Geometry check sheet. Reference: the model listing, model coordinates, mm. Face numbers are marked on the shaded views. A direction names the side the tool comes from. Coordinates: 2 decimals unless noted, no trailing zeros. Write each loop counter-clockwise with the first axis right and the second up, starting at its lowest first coordinate (ties: lowest second). Pieces come first, ordered by that corner, then holes. Notation, with made-up numbers: (17, -32.75) -> (51, -32.75) arc R16 ccw to (51, -27.75) -> close; hole circle Ø7 at (-3.75, 45). An arc over 180 degrees is marked (long way). Answer in a Markdown table with one row per item. Add a question column.
Q1. Release check for a two-part mould opening along Z. For the marked faces 1, 2, 3 and 4 record: pulls with the +Z half, pulls with the -Z half, needs draft (parallel to the pull), parting line crosses it, or undercut.
Q2. Tool access check on the marked faces 5 and 6. Record the directions out of +Z, -Z, +X, -X, +Y, -Y that give a thin tool (end or side, any length) a straight path to the whole face; none if there is none.
Q3. Section check B-B, the plane x = 11. Record the boundary of the cut face in (y, z), and give its area (3 significant figures).
Q4. Section check A-A, the plane z = -12. Record the boundary of the cut face in (x, y).
Q5. Gauge pin test, flat ends, axial feed: P1, Ø3, axis at x = -28.47, z = 35.745, coming from the +Y side; P2, Ø10, axis at x = -21, z = -12.5, coming from the +Y side; P3, Ø2, axis at x = -67.11, z = -42.11, coming from the +Y side. Record the tip position at first contact, or that the pin passes through.
Q6. Thickness scan on line 1 (Z direction, x = -28.47, y = 8) (3 decimals); line 2 (Z direction, x = -32.5, y = 26.75); line 3 (X direction, y = 24.5, z = 1.5). Record the ranges inside material, lowest first.
```python
from build123d import *

# Parameters (mm, degrees)
SKETCH1_W                 = 150
SKETCH1_H                 = 100
BOSS_EXTRUDE1_DEPTH       = 10
SKETCH2_R                 = 2.75
BOSS_EXTRUDE2_DEPTH       = 3
F_1_0MM_DOWEL_HOLE1_D     = 2.6
F_1_0MM_DOWEL_HOLE1_DEPTH = 10
F_1_0MM_DOWEL_HOLE1_TIP   = 0.781118805
FILLET1_R                 = 2
SKETCH5_W                 = 150
SKETCH5_H                 = 25
BOSS_EXTRUDE3_DEPTH       = 10
SKETCH7_W                 = 150
SKETCH7_H                 = 125
SKETCH7_W_2               = 136
SKETCH7_H_2               = 111
EXTRUDE_THIN1_DEPTH       = 20
CUT_EXTRUDE1_REACH        = 150.829
FILLET2_R                 = 15
FILLET3_R                 = 15
SKETCH9_R                 = 1.725
CUT_EXTRUDE2_DEPTH        = 6


with BuildPart() as part:
    # Sketch1 → Boss-Extrude1 (new body)
    with BuildSketch(Plane(origin=(0, 0, 0), x_dir=(1, 0, 0), z_dir=(0, 1, 0))):
        Rectangle(SKETCH1_W, SKETCH1_H)
    extrude(amount=BOSS_EXTRUDE1_DEPTH)

    # Sketch2 → Boss-Extrude2 (add)
    with BuildSketch(Plane(origin=(0, 10, 0), x_dir=(1, 0, 0), z_dir=(0, 1, 0))):
        with Locations(Location((28.47, 35.745, 0), (0, 0, 270))):
            Circle(SKETCH2_R)
        with Locations(Location((28.47, -35.745, 0), (0, 0, 90))):
            Circle(SKETCH2_R)
        with Locations(Location((-28.47, -35.745, 0), (0, 0, 270))):
            Circle(SKETCH2_R)
        with Locations(Location((-28.47, 35.745, 0), (0, 0, 90))):
            Circle(SKETCH2_R)
    extrude(amount=BOSS_EXTRUDE2_DEPTH)

    # Ø1.0mm Dowel Hole1
    with Locations(Plane(origin=(0, 13, 0), x_dir=(1, 0, 0), z_dir=(0, 1, 0))):
        with Locations((-28.47, 35.745), (28.47, 35.745), (28.47, -35.745), (-28.47, -35.745)):
            Hole(F_1_0MM_DOWEL_HOLE1_D / 2, depth=F_1_0MM_DOWEL_HOLE1_DEPTH)
            with Locations((0, 0, -(F_1_0MM_DOWEL_HOLE1_DEPTH + F_1_0MM_DOWEL_HOLE1_TIP / 2))):  # 118° drill point
                Cone(0, F_1_0MM_DOWEL_HOLE1_D / 2, F_1_0MM_DOWEL_HOLE1_TIP, mode=Mode.SUBTRACT)

    # Fillet1
    fillet1_edges = [part.edges().sort_by_distance(p)[0] for p in [
        (-28.47, 10, 32.995),
        (28.47, 10, -38.495),
        (28.47, 10, 38.495),
        (-28.47, 10, -32.995),
    ]]
    fillet(fillet1_edges, radius=FILLET1_R)

    # Sketch5 → Boss-Extrude3 (add)
    with BuildSketch(Plane.XZ):
        with Locations((0, 62.5)):
            Rectangle(SKETCH5_W, SKETCH5_H)
    extrude(amount=-BOSS_EXTRUDE3_DEPTH)

    # Sketch7 → Extrude-Thin1 (add)
    with BuildSketch(Plane(origin=(0, 10, 0), x_dir=(1, 0, 0), z_dir=(0, 1, 0))):
        with Locations((0, -12.5)):
            Rectangle(SKETCH7_W, SKETCH7_H)
        with Locations((0, -12.5)):
            Rectangle(SKETCH7_W_2, SKETCH7_H_2, mode=Mode.SUBTRACT)
    extrude(amount=EXTRUDE_THIN1_DEPTH)

    # Sketch8 → Cut-Extrude1 (cut, up to next)
    with BuildSketch(Plane.XY.offset(75), mode=Mode.PRIVATE) as cut_extrude1_sk1:
        with BuildLine():
            Line((-1.9, 30), (1.9, 30))
            Line((1.9, 30), (1.9, 24.2))
            ThreePointArc((1.9, 24.2), (1.607106781, 23.492893219), (0.9, 23.2))
            Line((0.9, 23.2), (-0.9, 23.2))
            ThreePointArc((-0.9, 23.2), (-1.607106781, 23.492893219), (-1.9, 24.2))
            Line((-1.9, 24.2), (-1.9, 30))
        make_face()
    cut_extrude1_tool1 = extrude(cut_extrude1_sk1.sketch, amount=-CUT_EXTRUDE1_REACH, mode=Mode.PRIVATE) & part.part
    add(cut_extrude1_tool1.solids().sort_by_distance((0, 26.653655, 75))[0], mode=Mode.SUBTRACT)

    # Fillet2
    fillet2_edges = [part.edges().sort_by_distance(p)[0] for p in [
        (-75, 15, 75),
        (75, 15, 75),
        (-75, 15, -50),
        (75, 15, -50),
    ]]
    fillet(fillet2_edges, radius=FILLET2_R)

    # Fillet3
    fillet3_edges = [part.edges().sort_by_distance(p)[0] for p in [
        (-68, 20, 68),
        (68, 20, 68),
        (68, 20, -43),
        (-68, 20, -43),
    ]]
    fillet(fillet3_edges, radius=FILLET3_R)

    # Sketch9 → Cut-Extrude2 (cut)
    with BuildSketch(Plane(origin=(0, 30, 0), x_dir=(1, 0, 0), z_dir=(0, 1, 0))):
        with Locations(Location((-67.106601718, 42.106601718, 0), (0, 0, 270))):
            Circle(SKETCH9_R)
        with Locations(Location((67.106601718, 42.106601718, 0), (0, 0, 90))):
            Circle(SKETCH9_R)
        with Locations(Location((67.106601718, -67.106601718, 0), (0, 0, 270))):
            Circle(SKETCH9_R)
        with Locations(Location((-67.106601718, -67.106601718, 0), (0, 0, 90))):
            Circle(SKETCH9_R)
    extrude(amount=-CUT_EXTRUDE2_DEPTH, mode=Mode.SUBTRACT)


solid = part.part
```
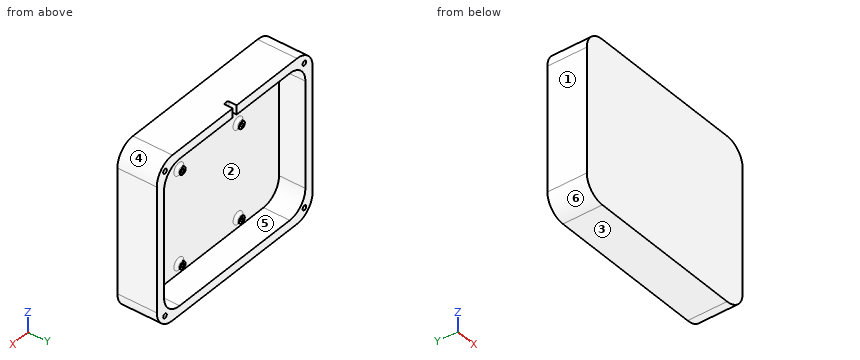
Calculated:
| question | item | result |
|---|---|---|
| 1 | face 1 | needs draft |
| 1 | face 2 | undercut |
| 1 | face 3 | pulls with the -Z half |
| 1 | face 4 | pulls with the +Z half |
| 2 | face 5 | +Y |
| 2 | face 6 | -Z, -X, +Y, -Y |
| 3 | outline | (0, -50) -> (30, -50) -> (30, -43) -> (10, -43) -> (10, 68) -> (30, 68) -> (30, 75) -> (0, 75) -> close |
| 3 | area | 1,530 mm² |
| 4 | outline | (-75, 0) -> (75, 0) -> (75, 30) -> (68, 30) -> (68, 10) -> (-68, 10) -> (-68, 30) -> (-75, 30) -> close |
| 5 | P1 | stops at y = 13 |
| 5 | P2 | stops at y = 10 |
| 5 | P3 | stops at y = 24 |
| 6 | line 1 | z = -50 to -37.045, -34.445 to 34.445, 37.045 to 75 |
| 6 | line 2 | z = -50 to -43, 68 to 75 |
| 6 | line 3 | x = -75 to -68, 68 to 75 |
